```python
from build123d import *
from build123d.topology import SkipClean

# Parameters (mm, degrees)
BASPROSKE_W         = 8
BASPROSKE_H         = 8.25
TOOTHCUT_DEPTH      = 15.146554351
TEETHCUTS_COUNT     = 10
TEETHCUTS_ANGLE     = 324
BORSKE_R            = 4.1
BORE_DEPTH          = 50.0000508
SKETCH_1_R          = 8.25
SKETCH_1_R_2        = 4.1
EXTRUDE_3_DEPTH     = 6
SKETCH_2_R          = 1.5
CUT_EXTRUDE_1_DEPTH = 16


with BuildPart() as part:
    # BasProSke → Base-Revolve (revolve)
    with BuildSketch(Plane(origin=(0, 0, 0), x_dir=(1, 0, 0), z_dir=(0, 1, 0)), mode=Mode.PRIVATE) as base_revolve_sk:
        with Locations((4, 4.125)):
            Rectangle(BASPROSKE_W, BASPROSKE_H)
    revolve(base_revolve_sk.sketch.rotate(Axis((-10, 0, 0), (1, 0, 0)), 180), axis=Axis((-10, 0, 0), (1, 0, 0)))

    # TooCutSke → ToothCut (cut, through all)
    with BuildSketch(Plane(origin=(0, 0, 0), x_dir=(0, 0, -1), z_dir=(1, 0, 0))):
        with BuildLine():
            ThreePointArc((0.931992048, 5.070305058), (0, 5.15525), (-0.931992048, 5.070305058))
            ThreePointArc((-0.931992048, 5.070305058), (-1.137854344, 6.727189108), (-2.264257491, 7.959609486))
            ThreePointArc((-2.264257491, 7.959609486), (0, 8.2754), (2.264257491, 7.959609486))
            ThreePointArc((2.264257491, 7.959609486), (1.137854344, 6.727189108), (0.931992048, 5.070305058))
        make_face()
    toothcut = extrude(amount=TOOTHCUT_DEPTH, mode=Mode.SUBTRACT)

    # TeethCuts: ToothCut ×10 about axis
    teethcuts_axis = Axis((-10, 0, 0), (1, 0, 0))
    for i in range(1, TEETHCUTS_COUNT):
        add(toothcut.rotate(teethcuts_axis, i * TEETHCUTS_ANGLE / (TEETHCUTS_COUNT - 1)), mode=Mode.SUBTRACT)

    # BorSke → Bore (cut, symmetric)
    with BuildSketch(Plane(origin=(0, 0, 0), x_dir=(0, 0, -1), z_dir=(1, 0, 0))):
        with Locations(Location((0, 0, 0), (0, 0, 180))):
            Circle(BORSKE_R)
    extrude(amount=BORE_DEPTH, both=True, mode=Mode.SUBTRACT)

    # Sketch 1 → Extrude 3 (add)
    with SkipClean():  # the faces are left unmerged after this step: merging them gives an invalid solid
        with BuildSketch(Plane.ZY):
            Circle(SKETCH_1_R)
            Circle(SKETCH_1_R_2, mode=Mode.SUBTRACT)
        extrude(amount=EXTRUDE_3_DEPTH)
    add(part.part.scale(1), mode=Mode.REPLACE)  # the faces are merged on a copy

    # Sketch 2 → Cut-Extrude 1 (cut)
    with BuildSketch(Plane(origin=(0, 0, 0), x_dir=(1, 0, 0), z_dir=(0, 1, 0))):
        with Locations(Location((-3, 0, 0), (0, 0, 270))):
            Circle(SKETCH_2_R)
    extrude(amount=-CUT_EXTRUDE_1_DEPTH, mode=Mode.SUBTRACT)


solid = part.part
```
Geometry: final body of the model. Coordinates: model frame, mm. Give positions to 0.01 mm unless a question says otherwise; leave off trailing zeros. Order: outer loops, then holes, each group sorted by start corner. A loop starts at its lowest first (then second) coordinate and runs counter-clockwise, first axis right, second up. Notation, with made-up numbers: M 69,53.25 L 110,53.25 A30 cw 110,75.25 Z; hole C 2,33 d10. An arc over 180 degrees is marked long. Answer as CSV lines item,"result". Start each with the question number.
1) Cut plane C-C (z = -2.5). Output: boundary loops of the cut face in (x, y), then the cut area to 3 significant figures.
2) Cut plane B-B (y = 1.75). Output: boundary loops of the cut face in (x, z), then the cut area to 3 significant figures.
3) Cut plane A-A (z = 0). Output: boundary loops of the cut face in (x, y).
4) First-contact query: P1, Ø1.9, axis at y = 3, z = -6, coming from the +X side; P2, Ø3, axis at x = 5, y = 3, coming from the -Z side; P3, Ø1.5, axis at x = 5.5, y = -6, coming from the -Z side; P4, Ø1, axis at x = 4, z = 5.5, coming from the -Y side. Flat tips, straight axial feed; report the tip coordinate or a pass-through.
5) Cut plane D-D (x = -3). Output: boundary loops of the cut face in (y, z).
6) Line query: line 1 (Y direction, x = 5.75, z = 0); line 2 (Z direction, x = -3.5, y = 0); line 3 (X direction, y = -5.4, z = 0). Output: solid intervals per line, ascending. Write a range as from..to.
Findings below:
1,outline,"M -6,-7.86 L 8,-7.86 L 8,-4.95 L 0,-4.95 L 0,-4.51 L 8,-4.51 L 8,-3.25 L -6,-3.25 Z; M -6,3.25 L 8,3.25 L 8,4.51 L 0,4.51 L 0,4.95 L 8,4.95 L 8,7.86 L -6,7.86 Z"
1,area,"122 mm²"
2,outline,"M -6,-8.06 L 0,-8.06 L 0,-4.85 L 8,-4.85 L 8,-3.71 L -6,-3.71 Z; M -6,3.71 L 8,3.71 L 8,4.85 L 0,4.85 L 0,8.06 L -6,8.06 Z"
2,area,"70.5 mm²"
3,outline,"M -6,-8.25 L -4.5,-8.25 L -4.5,-4.1 L -6,-4.1 Z; M -6,4.1 L 8,4.1 L 8,5.16 L 0,5.16 L 0,8.25 L -6,8.25 Z; M -1.5,-8.25 L 0,-8.25 L 0,-5.16 L 8,-5.16 L 8,-4.1 L -1.5,-4.1 Z"
4,P1,"stops at x = 8"
4,P2,"stops at z = -6.84"
4,P3,"stops at z = -3.09"
4,P4,"stops at y = -5.12"
5,outline,"M -8.11,-1.5 A8.25 ccw long -8.11,1.5 L -3.82,1.5 A4.1 cw long -3.82,-1.5 Z"
6,line 1,"y = -5.16..-4.1, 4.1..5.16"
6,line 2,"z = -8.25..-4.1, 4.1..8.25"
6,line 3,"x = -6..-4.5, -1.5..0"
